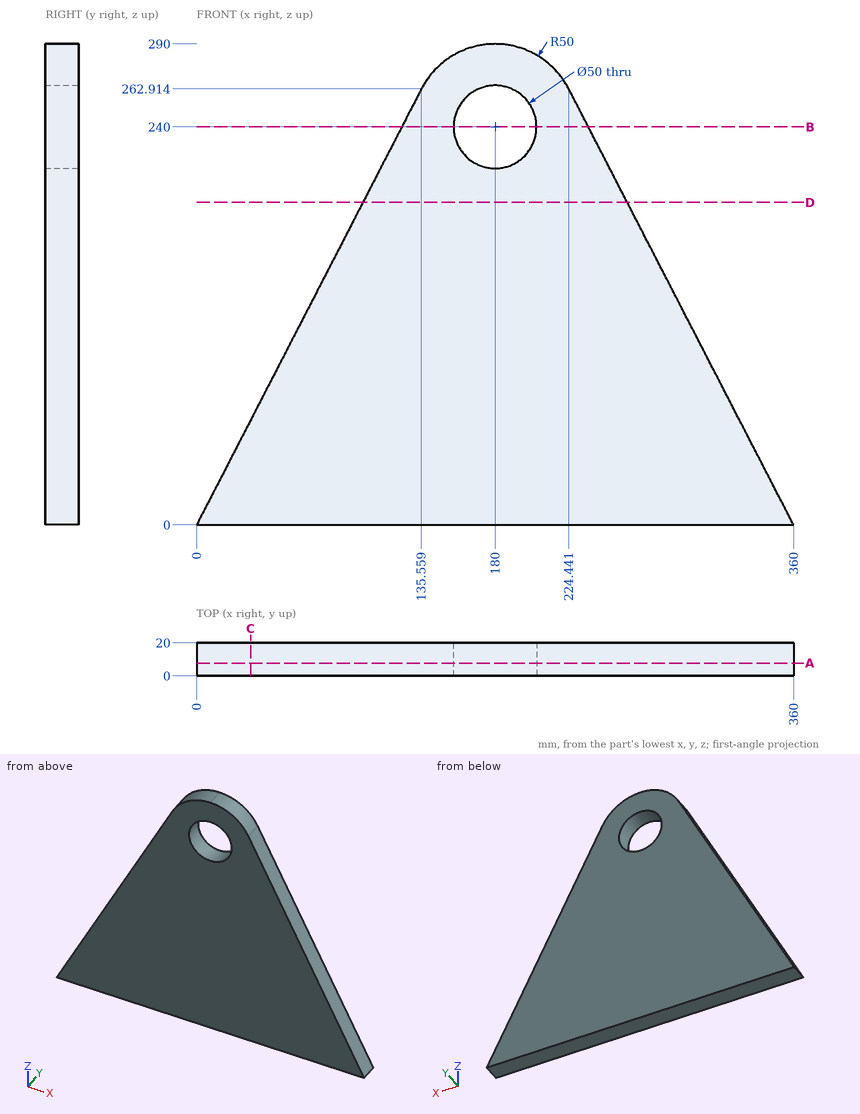
Job drawing, mm, ordinate dimensions from the low corner. One solid piece. Round coordinates to 2 decimals unless told otherwise and drop trailing zeros. Write each loop counter-clockwise with the first axis right and the second up, starting at its lowest first coordinate (ties: lowest second). Pieces come first, ordered by that corner, then holes. Notation, with made-up numbers: (-25, 29) -> (-21, 29) arc R32 ccw to (-21, 63) -> close; hole circle Ø1 at (9.5, 70.25). An arc over 180 degrees is marked (long way). Answer as a JSON object with one key per item and string values.
(1) Band-saw the part on B-B, the plane z = 240. List the corners of the cut face in (x, y) (1 decimal), then the cut area to 3 significant figures.
Reported:
{"outline": "(123.7, 0) -> (155, 0) -> (155, 20) -> (123.7, 20) -> close; (205, 0) -> (236.3, 0) -> (236.3, 20) -> (205, 20) -> close", "area": "1,250 mm^2"}
(2) Band-saw the part on A-A, the plane y = 7.75. List the corners of the cut face in (x, z).
Reported:
{"outline": "(0, 0) -> (360, 0) -> (224.44, 262.91) arc R50 ccw to (180, 290) arc R50 ccw to (135.56, 262.91) -> close; hole circle Ø50 at (180, 240)"}
(3) Band-saw the part on D-D, the plane z = 194.5. List the corners of the cut face in (x, y) (1 decimal), then the cut area to 3 significant figures.
Reported:
{"outline": "(100.3, 0) -> (259.7, 0) -> (259.7, 20) -> (100.3, 20) -> close", "area": "3,190 mm^2"}
(4) Probe probe 1 along Z at (x, y) = (163, 17.75); probe 2 along X at (y, z) = (4, 181) (1 decimal); probe 3 along X at (y, z) = (8.25, 185) (1 decimal). List the from-to ranges inside material, lowest first. Write a range as [from, to].
Reported:
{"probe 1": "z = [0, 221.67], [258.33, 287.02]", "probe 2": "x = [93.3, 266.7]", "probe 3": "x = [95.4, 264.6]"}
(5) Band-saw the part on C-C, the plane x = 32.5. List the corners of the cut face in (y, z).
Reported:
{"outline": "(0, 0) -> (20, 0) -> (20, 63.03) -> (0, 63.03) -> close"}
(6) Pin check, flat tips, straight feed: P1, Ø5, axis at x = 226.5, y = 9.5, coming from the +Z side; P2, Ø2, axis at y = 3, z = 210.5, coming from the -X side; P3, Ø6, axis at x = 58, y = 9.5, coming from the +Z side (1 decimal); P4, Ø4, axis at x = 67.5, y = 6, coming from the -Z side. Stop position of each tip, or through.
Reported:
{"P1": "stops at z = 263.75", "P2": "stops at x = 108.02", "P3": "stops at z = 118.3", "P4": "stops at z = 0"}
